CAD build for the part. Positions are in the model's coordinates, mm. Face numbers are marked on the shaded views. Coordinates: 2 decimals unless noted, no trailing zeros. Write each loop counter-clockwise with the first axis right and the second up, starting at its lowest first coordinate (ties: lowest second). Pieces come first, ordered by that corner, then holes. Notation, with made-up numbers: (-32.75, 35) - (15.25, 35) arc R15 cw to (15.25, 44) - close; hole circle Ø1 at (-34, -31.75). An arc over 180 degrees is marked (long way). Answer in a Markdown table with one row per item. Add a question column.
Q1. Band-saw the part on A-A (x = -52.5). List the corners of the cut face in (y, z), and give its area (3 significant figures).
Q2. Band-saw the part on B-B (y = 15). List the corners of the cut face in (x, z).
Q3. Drill centre lines: line 1 along Y through (x, z) = (-52.5, 21.5); line 2 along Y through (x, z) = (-37.5, 22); line 3 along X through (y, z) = (13.5, 19.5). Where is each one in solid material? Low to high. Write a range as from..to.
Q4. Band-saw the part on C-C (z = 16). List the corners of the cut face in (x, y).
Q5. Two-plate mould, pull along X, no slides. Class the marked faces 1, 2, 3 and 4: +X half, -X half, draft (parallel to the pull), parting line (faces both ways), or undercut.
```python
from build123d import *

# Parameters (mm, degrees)
F1_DEPTH = 25
F2_R     = 6
F2_R_2   = 8.25
F2_R_3   = 8
F3_DEPTH = 20
F5_DEPTH = 25.001
F6_W     = 34.932942614
F6_H     = 15
F7_DEPTH = 34.2048565129


with BuildPart() as f1:
    # F0 (on Top) → F1 (new body)
    with BuildSketch(Plane.XY):
        with BuildLine():
            Line((-58.75, -42.5), (58.75, -42.5))
            ThreePointArc((58.75, -42.5), (62.2855339059, -41.0355339059), (63.75, -37.5))
            Line((63.75, -37.5), (63.75, 37.5))
            ThreePointArc((63.75, 37.5), (62.2855339059, 41.0355339059), (58.75, 42.5))
            Line((58.75, 42.5), (-58.75, 42.5))
            ThreePointArc((-58.75, 42.5), (-62.2855339059, 41.0355339059), (-63.75, 37.5))
            Line((-63.75, 37.5), (-63.75, -37.5))
            ThreePointArc((-63.75, -37.5), (-62.2855339059, -41.0355339059), (-58.75, -42.5))
        make_face()
    extrude(amount=F1_DEPTH)

    # F2 (on face) → F3 (cut)
    with BuildSketch(Plane.XY.offset(25)):
        with Locations((-52.5, 15)):
            Circle(F2_R)
        with Locations((-52.5, 0)):
            Circle(F2_R)
        with Locations((-52.5, -15)):
            Circle(F2_R)
        with Locations((-37.5, 30)):
            Circle(F2_R)
        with Locations((-37.5, 15)):
            Circle(F2_R)
        with Locations((-37.5, 0)):
            Circle(F2_R)
        with Locations((-37.5, -15)):
            Circle(F2_R)
        with Locations((-37.5, -30)):
            Circle(F2_R)
        with Locations((-22.5, 30)):
            Circle(F2_R)
        with Locations((-22.5, 15)):
            Circle(F2_R)
        with Locations((-22.5, 0)):
            Circle(F2_R)
        with Locations((-22.5, -15)):
            Circle(F2_R)
        with Locations((-22.5, -30)):
            Circle(F2_R)
        with Locations((-7.5, 30)):
            Circle(F2_R)
        with Locations((-7.5, 15)):
            Circle(F2_R)
        with Locations((-7.5, 0)):
            Circle(F2_R)
        with Locations((-7.5, -15)):
            Circle(F2_R)
        with Locations((-7.5, -30)):
            Circle(F2_R)
        with Locations((7.5, 30)):
            Circle(F2_R)
        with Locations((7.5, 15)):
            Circle(F2_R)
        with Locations((7.5, 0)):
            Circle(F2_R)
        with Locations((7.5, -15)):
            Circle(F2_R)
        with Locations((7.5, -30)):
            Circle(F2_R)
        with Locations((22.5, 30)):
            Circle(F2_R)
        with Locations((22.5, 15)):
            Circle(F2_R)
        with Locations((22.5, 0)):
            Circle(F2_R)
        with Locations((22.5, -15)):
            Circle(F2_R)
        with Locations((22.5, -30)):
            Circle(F2_R)
        with Locations((37.5, 30)):
            Circle(F2_R)
        with Locations((37.5, 15)):
            Circle(F2_R)
        with Locations((37.5, 0)):
            Circle(F2_R)
        with Locations((37.5, -15)):
            Circle(F2_R)
        with Locations((37.5, -30)):
            Circle(F2_R)
        with Locations((52.5, 15)):
            Circle(F2_R)
        with Locations((52.5, 0)):
            Circle(F2_R)
        with Locations((52.5, -15)):
            Circle(F2_R)
        with Locations((-52.5, 30)):
            Circle(F2_R_2)
        with Locations((-52.5, -30)):
            Circle(F2_R_3)
        with Locations((52.5, 30)):
            Circle(F2_R_3)
        with Locations((52.5, -30)):
            Circle(F2_R_3)
    extrude(amount=-F3_DEPTH, mode=Mode.SUBTRACT)

    # F4 (on face) → F5 (cut, through all)
    with BuildSketch(Plane.XY.offset(25)):
        Polygon((69.5764049888, -59.449698776), (69.5764049888, 48.7273074687), (-29.5461434871, 48.7273074687), (-29.5461434871, 7.567057386), (-74.2632374167, 7.567057386), (-74.2632374167, 4.9460288137), (-74.2632374167, -59.449698776), align=None)
    extrude(amount=-F5_DEPTH, mode=Mode.SUBTRACT)

    # F6 (on face) → F7 (cut, through all)
    with BuildSketch(Plane.YZ.offset(-29.5461434871)):
        with Locations((25.033528693, 7.5)):
            Rectangle(F6_W, F6_H)
    extrude(amount=-F7_DEPTH, mode=Mode.SUBTRACT)


solid = f1.part
```
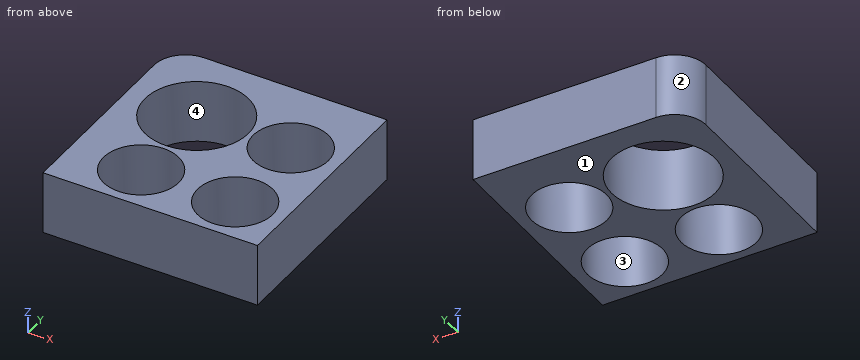
Checked values:
| question | item | result |
|---|---|---|
| 1 | outline | (7.57, 15) - (9, 15) - (9, 25) - (7.57, 25) - close; (21, 15) - (21.75, 15) - (21.75, 25) - (21, 25) - close; (38.25, 15) - (42.5, 15) - (42.5, 25) - (38.25, 25) - close |
| 1 | area | 64.3 mm² |
| 2 | outline | (-63.75, 15) - (-58.5, 15) - (-58.5, 25) - (-63.75, 25) - close; (-46.5, 15) - (-43.5, 15) - (-43.5, 25) - (-46.5, 25) - close; (-31.5, 15) - (-29.55, 15) - (-29.55, 25) - (-31.5, 25) - close |
| 3 | line 1 | y = 7.57..9, 21..21.75, 38.25..42.5 |
| 3 | line 2 | y = 7.57..9, 21..24, 36..42.5 |
| 3 | line 3 | x = -63.75..-58.31, -46.69..-43.31, -31.69..-29.55 |
| 4 | outline | (-63.75, 7.57) - (-29.55, 7.57) - (-29.55, 42.5) - (-58.75, 42.5) arc R5 ccw to (-63.75, 37.5) - close; hole circle Ø16.5 at (-52.5, 30); hole circle Ø12 at (-52.5, 15); hole circle Ø12 at (-37.5, 15); hole circle Ø12 at (-37.5, 30) |
| 5 | face 1 | draft |
| 5 | face 2 | -X half |
| 5 | face 3 | undercut |
| 5 | face 4 | undercut |
